Source: CAD feature listing. Evaluate the final solid. Frame: model axes, mm. A direction names the side the tool comes from. Coordinates: 2 decimals unless noted, no trailing zeros. Order: outer loops, then holes, each group sorted by start corner. A loop starts at its lowest first (then second) coordinate and runs counter-clockwise, first axis right, second up.
Item 1: Section A-A on x = 10. Return the cut outline in (y, z).
Item 2: Mould query, pull axis X, two halves, no side actions, for faces 3 (the flat face through (17, 0, 3)), 4 (the cylindrical face through (33.706, 9.658, 15.056)), 5 (the flat face through (-21.41, 9, 2)). Classes: released by +X, released by -X, zero draft, split by the parting line, or undercut.
Item 3: Ray query, line 1 (Z direction, x = 27, y = 18.75); line 2 (Z direction, x = 2.5, y = 1.75); line 3 (X direction, y = 13.75, z = 17). Return the intervals inside material, ascending.
Item 4: Section B-B on z = 12. Return the cut outline in (x, y).
Item 5: Reachability of faces 1 (the flat face through (17, 10, 10.643)), 2 (the flat face through (17, 19.05, 3)) from +Z, -Z, +X, -X, +Y, -Y: full face, straight path, thin tool, end or side. Return the list, or none.
Item 6: Section C-C on y = 5. Return the cut outline in (x, z).
Autodesk Inventor part; units mm, degrees
ref_plane "YZ Plane" through (0, 0, 0) normal (1, 0, 0) x (0, 1, 0)
ref_plane "XZ Plane" through (0, 0, 0) normal (0, 1, 0) x (-1, 0, 0)
ref_plane "XY Plane" through (0, 0, 0) normal (0, 0, 1) x (1, 0, 0)
sketch "Sketch1" plane through (0, 0, 0) normal (0, 1, 0) x (-1, 0, 0)
  line L0 (21.4105, 40.3607) -> (-54.7895, 40.3607)
  line L1 (-54.7895, 40.3607) -> (-54.7895, -35.8393)
  line L2 (-54.7895, -35.8393) -> (21.4105, -35.8393)
  line L3 (21.4105, -35.8393) -> (21.4105, 40.3607)
  point P0 (0, 0)
  dimension "d0" = 76.2
  dimension "d1" = 76.2
extrude "Extrusion1" add sketch "Sketch1" along normal blind 19.05
sketch "Sketch2" plane through (0, 19.05, 0) normal (0, 1, 0) x (1, 0, 0)
  arc A0 (3.9895, -10.6427) -> (3.9895, -19.2787) centre (3.9895, -14.9607) ccw
  line L0 (-21.4105, 35.8393) -> (-21.4105, -40.3607)
  line L1 (-21.4105, -40.3607) -> (54.7895, -40.3607)
  arc A1 (29.3895, -19.2787) -> (29.3895, -10.6427) centre (29.3895, -14.9607) ccw
  line L2 (54.7895, -40.3607) -> (54.7895, 35.8393)
  line L3 (3.9895, -19.2787) -> (29.3895, -19.2787)
  line L4 (3.9895, -10.6427) -> (29.3895, -10.6427)
  point P0 (0, 0)
  dimension "d4" = 8.636
  dimension "d5" = 25.4
  dimension "d6" = 25.4
  dimension "d7" = 8.636
  dimension "d8" = 25.4
  dimension "d9" = 25.4
extrude "Extrusion2" cut sketch "Sketch2" against normal through all
sketch "Sketch3" plane through (0, 19.05, 0) normal (0, 1, 0) x (1, 0, 0)
  arc A0 (3.9895, 14.7573) -> (3.9895, 6.1213) centre (3.9895, 10.4393) ccw
  line L0 (-21.4105, 35.8393) -> (-21.4105, -40.3607)
  line L1 (54.7895, 35.8393) -> (-21.4105, 35.8393)
  arc A1 (29.3895, 6.1213) -> (29.3895, 14.7573) centre (29.3895, 10.4393) ccw
  line L2 (54.7895, -40.3607) -> (54.7895, 35.8393)
  line L3 (3.9895, 6.1213) -> (29.3895, 6.1213)
  line L4 (3.9895, 14.7573) -> (29.3895, 14.7573)
  point P0 (0, 0)
  dimension "d12" = 8.636
  dimension "d13" = 25.4
  dimension "d14" = 25.4
  dimension "d15" = 8.636
  dimension "d16" = 25.4
  dimension "d17" = 25.4
extrude "Extrusion3" add sketch "Sketch3" against normal through all
sketch "Sketch4" plane through (0, 19.05, 0) normal (0, 1, 0) x (1, 0, 0)
  arc A0 (3.9895, 14.7573) -> (3.9895, 6.1213) centre (3.9895, 10.4393) ccw
  line L0 (54.7895, 35.8393) -> (-21.4105, 35.8393)
  line L1 (-21.4105, 35.8393) -> (-21.4105, -40.3607)
  arc A1 (29.3895, 6.1213) -> (29.3895, 14.7573) centre (29.3895, 10.4393) ccw
  line L2 (54.7895, -40.3607) -> (54.7895, 35.8393)
  line L3 (3.9895, 6.1213) -> (29.3895, 6.1213)
  line L4 (29.3895, 14.7573) -> (3.9895, 14.7573)
  point P0 (0, 0)
  dimension "d20" = 8.636
  dimension "d21" = 25.4
  dimension "d22" = 25.4
  dimension "d23" = 8.636
  dimension "d24" = 25.4
  dimension "d25" = 25.4
extrude "Extrusion4" cut sketch "Sketch4" against normal blind 19.05
properties part number "slotted riser 1"
Answer list:
1. outline: (0, -35.84) - (19.05, -35.84) - (19.05, -14.76) - (0, -14.76) - close; (0, -6.12) - (19.05, -6.12) - (19.05, 10.64) - (0, 10.64) - close; (0, 19.28) - (19.05, 19.28) - (19.05, 40.36) - (0, 40.36) - close
2. face 3: zero draft
2. face 4: undercut
2. face 5: released by -X
3. line 1: z = -35.84 to -14.76, -6.12 to 10.64, 19.28 to 40.36
3. line 2: z = -35.84 to -14.49, -6.39 to 10.91, 19.01 to 40.36
3. line 3: x = -21.41 to 0.18, 33.2 to 54.79
4. outline: (-21.41, 0) - (0.85, 0) - (0.85, 19.05) - (-21.41, 19.05) - close; (32.53, 0) - (54.79, 0) - (54.79, 19.05) - (32.53, 19.05) - close
5. face 1: +Y, -Y
5. face 2: +Z, -Z, +X, -X, +Y
6. outline: (-21.41, -35.84) - (54.79, -35.84) - (54.79, 40.36) - (-21.41, 40.36) - close; hole (3.99, -14.76) - (29.39, -14.76) arc R4.32 ccw to (29.39, -6.12) - (3.99, -6.12) arc R4.32 ccw to start; hole (3.99, 10.64) - (29.39, 10.64) arc R4.32 ccw to (29.39, 19.28) - (3.99, 19.28) arc R4.32 ccw to start
